from build123d import *

# Parameters (mm, degrees)
CROQUIS1_W              = 5
CROQUIS1_H              = 3
SALIENTE_EXTRUIR1_DEPTH = 15
SALIENTE_EXTRUIR2_DEPTH = 10


with BuildPart() as part:
    # Croquis1 → Saliente-Extruir1 (new body)
    with BuildSketch(Plane(origin=(0, 0, 0), x_dir=(1, 0, 0), z_dir=(0, 1, 0))):
        with BuildLine():
            Line((-2.75, -2), (2.75, -2))
            ThreePointArc((2.75, -2), (2.926776695, -1.926776695), (3, -1.75))
            Line((3, -1.75), (3, 1.75))
            ThreePointArc((3, 1.75), (2.926776695, 1.926776695), (2.75, 2))
            Line((2.75, 2), (-2.75, 2))
            ThreePointArc((-2.75, 2), (-2.926776695, 1.926776695), (-3, 1.75))
            Line((-3, 1.75), (-3, -1.75))
            ThreePointArc((-3, -1.75), (-2.926776695, -1.926776695), (-2.75, -2))
        make_face()
        Rectangle(CROQUIS1_W, CROQUIS1_H, mode=Mode.SUBTRACT)
    extrude(amount=SALIENTE_EXTRUIR1_DEPTH)

    # Croquis2 → Saliente-Extruir2 (add)
    with BuildSketch(Plane(origin=(0, 15, 0), x_dir=(1, 0, 0), z_dir=(0, 1, 0))):
        with BuildLine():
            Line((-3.25, 0), (-15, 0))
            Line((-15, 0), (0, -3.25))
            ThreePointArc((0, -3.25), (2.298097039, -2.298097039), (3.25, 0))
            Line((3.25, 0), (15, 0))
            Line((15, 0), (0, 3.25))
            ThreePointArc((0, 3.25), (-2.298097039, 2.298097039), (-3.25, 0))
        make_face()
    extrude(amount=SALIENTE_EXTRUIR2_DEPTH)


solid = part.part
Source: CAD feature listing. Evaluate the final solid. Frame: model axes, mm. A direction names the side the tool comes from. Coordinates: 2 decimals unless noted, no trailing zeros. Loops run counter-clockwise (first coordinate to the right, second up) from the corner with the lowest first, then second, coordinate; pieces in that order, holes last. Notation, with made-up numbers: (-0.75, 16) - (14.25, 16) arc R24 cw to (14.25, 28) - close; hole circle Ø7 at (28.25, 15). An arc over 180 degrees is marked (long way). One line per item, written item: value. Start each with the question number.
1. Contact query for flat-ended pins moving along their axis: P1, Ø2.5, axis at y = 5, z = -0.5, coming from the +X side; P2, Ø1, axis at x = 11.5, z = 1, coming from the +Y side; P3, Ø3, axis at x = 6, y = 20.5, coming from the +Z side; P4, Ø1.6, axis at x = 0.5, y = 6.5, coming from the -Z side. Output: stop coordinate, or through.
2. Mould query, pull axis X, two halves, no side actions, for faces 1 (the flat face through (6, 15, -1)), 2 (the flat face through (7.605, 19.93, -1.602)), 3 (the flat face through (2.5, 7, 0)). Classes: pulls with the +X half, pulls with the -X half, needs draft (parallel to the pull), parting line crosses it, or undercut.
3. Section A-A (y = 8.25). Return the cut outline in (x, z).
4. Section D-D (x = -8). Return the cut outline in (y, z), and give its area (3 significant figures).
5. Ray query, L1, parallel to Z at x = 2, y = 14.5; L2, parallel to X at y = 1.5, z = 0.75; L3, parallel to Y at x = 3.5, z = -0.5. Return the intervals inside material, ascending.
6. Section C-C (z = -0.5). Return the cut outline in (x, y), and give its area (3 significant figures).
7. Section B-B (x = 1.25). Return the cut outline in (y, z), and give its area (3 significant figures).
8. Set-up query: faces 4 (the flat face through (9, 20, 0)), 5 (the flat face through (-2.5, 7, 0)), 6 (the flat face through (3, 7, 0)), 7 (the flat face through (-5, 15, 1)). Return all of +Z, -Z, +X, -X, +Y, -Y with unobstructed straight access to the full face (end or side cutting, diameter ignored); none if empty.
Verdict:
1. P1: stops at x = 3
1. P2: passes through
1. P3: stops at z = 0
1. P4: stops at z = -2
2. face 1: needs draft
2. face 2: pulls with the +X half
2. face 3: undercut
3. outline: (-3, -1.75) arc R0.25 ccw to (-2.75, -2) - (2.75, -2) arc R0.25 ccw to (3, -1.75) - (3, 1.75) arc R0.25 ccw to (2.75, 2) - (-2.75, 2) arc R0.25 ccw to (-3, 1.75) - close; hole (-2.5, -1.5) - (2.5, -1.5) - (2.5, 1.5) - (-2.5, 1.5) - close
4. outline: (15, 0) - (25, 0) - (25, 1.52) - (15, 1.52) - close
4. area: 15.2 mm2
5. L1: z = -2 to -1.5, 1.5 to 2
5. L2: x = -3 to -2.5, 2.5 to 3
5. L3: y = 15 to 25
6. outline: (-3.21, 15) - (-3, 15) - (-3, 0) - (-2.5, 0) - (-2.5, 15) - (2.5, 15) - (2.5, 0) - (3, 0) - (3, 15) - (12.69, 15) - (12.69, 25) - (-3.21, 25) - close
6. area: 174 mm2
7. outline: (0, -2) - (15, -2) - (15, -2.98) - (25, -2.98) - (25, 3) - (15, 3) - (15, 2) - (0, 2) - (0, 1.5) - (15, 1.5) - (15, -1.5) - (0, -1.5) - close
7. area: 74.8 mm2
8. face 4: +Z, +X, +Y, -Y
8. face 5: -Y
8. face 6: +Z, -Z, +X, -Y
8. face 7: +Z, -X, -Y
